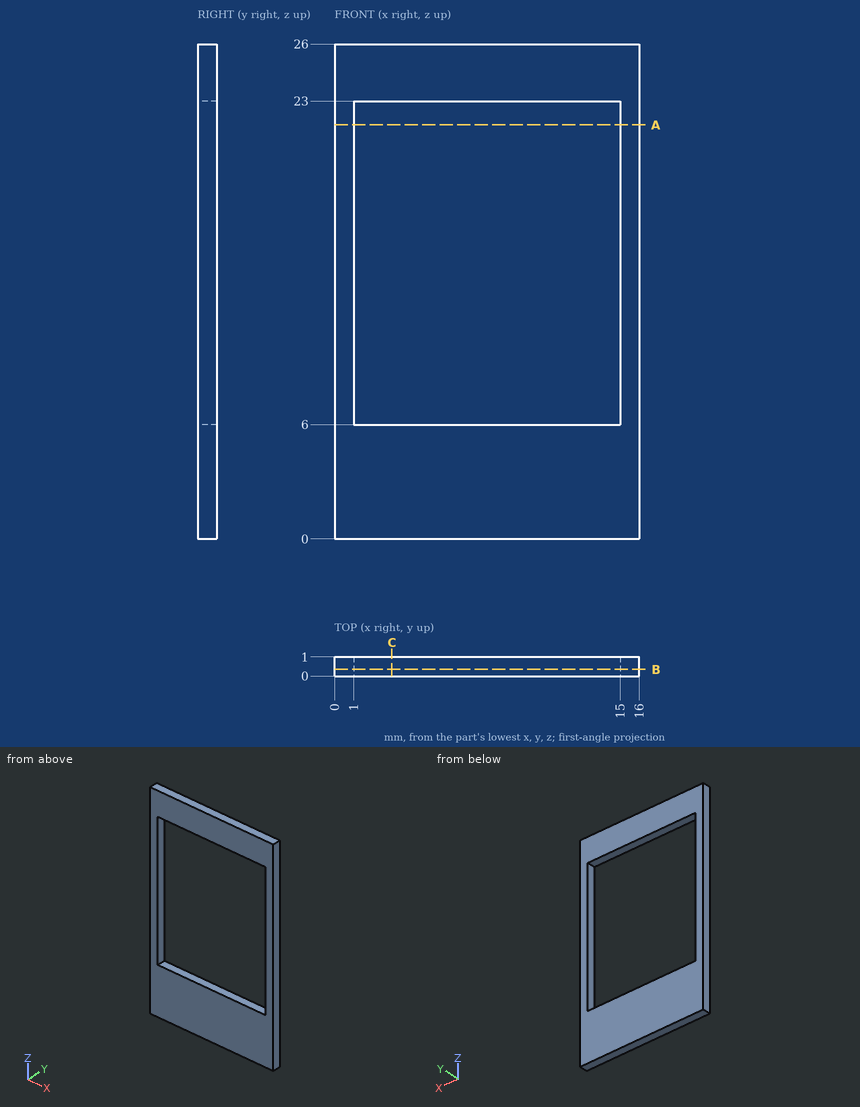
Geometry: see drawing. Coordinates: mm, zero at the bounding-box minimum. Round coordinates to 2 decimals unless told otherwise and drop trailing zeros. Loops run counter-clockwise (first coordinate to the right, second up) from the corner with the lowest first, then second, coordinate; pieces in that order, holes last. Notation, with made-up numbers: M 13,25.25 L 26,25.25 A14 ccw 26,30.25 Z; hole C 53,-1.5 d5. An arc over 180 degrees is marked long. Use a Markdown table: item, result. Add a question column.
1. Ray query, line 1 along Z through (x, y) = (6.5, 0.5); line 2 along X through (y, z) = (0.4, 10.5). Return the intervals inside material, ascending. Write a range as [from, to].
2. Cut plane A-A, the plane z = 21.75. Output: boundary loops of the cut face in (x, y).
3. Cut plane B-B, the plane y = 0.35. Output: boundary loops of the cut face in (x, z).
4. Cut plane C-C, the plane x = 3. Output: boundary loops of the cut face in (y, z), and give its area (3 significant figures).
Solution:
| question | item | result |
|---|---|---|
| 1 | line 1 | z = [0, 6], [23, 26] |
| 1 | line 2 | x = [0, 1], [15, 16] |
| 2 | outline | M 0,0 L 1,0 L 1,1 L 0,1 Z; M 15,0 L 16,0 L 16,1 L 15,1 Z |
| 3 | outline | M 0,0 L 16,0 L 16,26 L 0,26 Z; hole M 1,6 L 15,6 L 15,23 L 1,23 Z |
| 4 | outline | M 0,0 L 1,0 L 1,6 L 0,6 Z; M 0,23 L 1,23 L 1,26 L 0,26 Z |
| 4 | area | 9.00 mm2 |
